Design review of the part shown in the three views and the two pictorial views. Dimensions are in mm from the part's minimum x, y and z. Give positions to 0.01 mm unless a question says otherwise; leave off trailing zeros. Order: outer loops, then holes, each group sorted by start corner. A loop starts at its lowest first (then second) coordinate and runs counter-clockwise, first axis right, second up. Notation, with made-up numbers: M 19,-19.75 L 58,-19.75 A27 cw 58,0.25 Z; hole C 39,24 d1. An arc over 180 degrees is marked long. Answer as a JSON object with one key per item and string values.
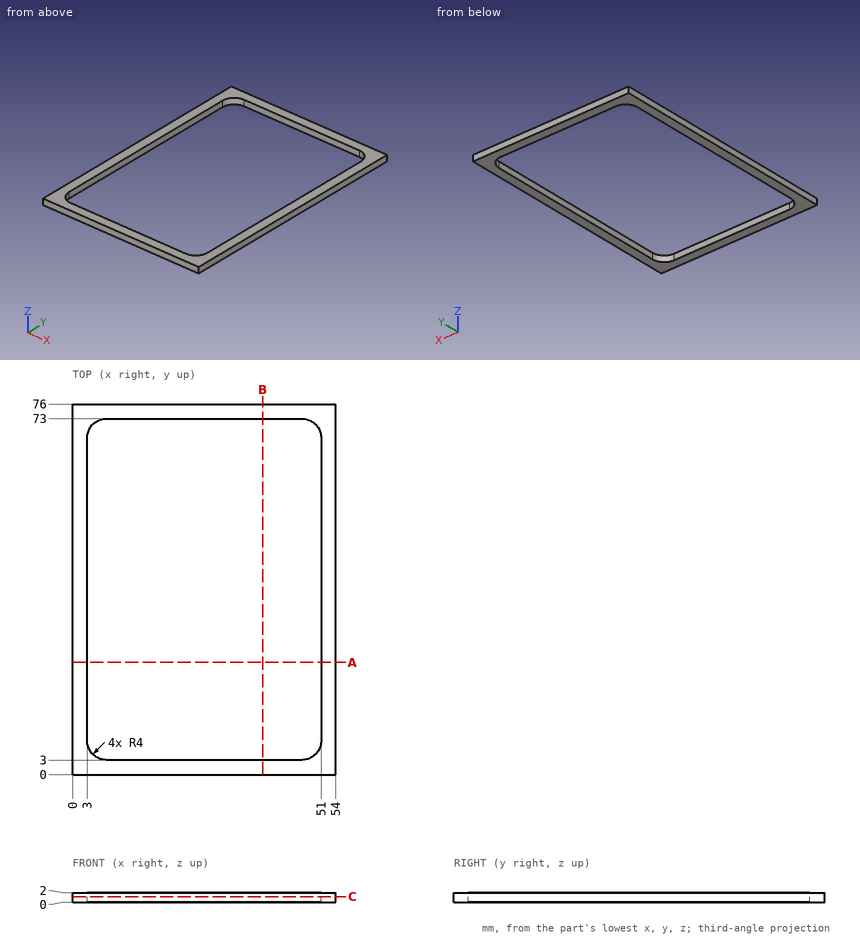
(1) We need section C-C (z = 1.2). Write out the cut boundary in (x, y).
Checked values:
{"outline": "M 0,0 L 54,0 L 54,76 L 0,76 Z; hole M 3,7 A4 ccw 7,3 L 47,3 A4 ccw 51,7 L 51,69 A4 ccw 47,73 L 7,73 A4 ccw 3,69 Z"}
(2) We need section A-A (y = 23). Write out the cut boundary in (x, z).
Checked values:
{"outline": "M 0,0 L 3,0 L 3,2 L 0,2 Z; M 51,0 L 54,0 L 54,2 L 51,2 Z"}
(3) We need section B-B (x = 39). Write out the cut boundary in (y, z).
Checked values:
{"outline": "M 0,0 L 3,0 L 3,2 L 0,2 Z; M 73,0 L 76,0 L 76,2 L 73,2 Z"}
(4) To check wall thickness, follow L1, parallel to Y at x = 40, z = 1.6; L2, parallel to X at y = 35, z = 0.25; L3, parallel to Y at x = 5, z = 0.8. State the ranges of each line that lie inside material, in increasing order. Write a range as from..to.
Checked values:
{"L1": "y = 0..3, 73..76", "L2": "x = 0..3, 51..54", "L3": "y = 0..3.54, 72.46..76"}
